Can you work these out from the model? Positions are in its coordinate system, mm. A direction names the side the tool comes from. Give positions to 0.01 mm unless a question says otherwise; leave off trailing zeros. Order: outer loops, then holes, each group sorted by start corner. A loop starts at its lowest first (then second) coordinate and runs counter-clockwise, first axis right, second up. Notation, with made-up numbers: (-30, 76) - (-3, 76) arc R25 cw to (-3, 93) - close; hole circle Ø11 at (45.5, 35.25). An arc over 180 degrees is marked (long way). Answer as a JSON object with one key per item and string values.
```python
from build123d import *

# Parameters (mm, degrees)
F0_W     = 40
F0_H     = 16
F0_W_2   = 32
F0_H_2   = 8
F1_DEPTH = 2.5
F2_R     = 2
F4_DEPTH = 12.5


with BuildPart() as f1:
    # F0 (on Top) → F1 (new body, symmetric)
    with BuildSketch(Plane.XY):
        Rectangle(F0_W, F0_H)
        Rectangle(F0_W_2, F0_H_2, mode=Mode.SUBTRACT)
    extrude(amount=F1_DEPTH, both=True)

    # F2
    f2_edges = [f1.edges().sort_by_distance(p)[0] for p in [
        (-20, 8, 0),
        (-20, -8, 0),
        (20, -8, 0),
        (20, 8, 0),
    ]]
    fillet(f2_edges, radius=F2_R)

    # F3 (on face) → F4 (cut, symmetric)
    with BuildSketch(Plane.XY.offset(2.5)):
        Polygon((16, 0), (16, -2.256422), (20, 0.861545), (20, 2.871813), align=None)
    extrude(amount=F4_DEPTH, both=True, mode=Mode.SUBTRACT)


solid = f1.part
```
Q1. Which directions (+Z, -Z, +X, -X, +Y, -Y) give clear straight access to the entire face, cutting with the end or side of a thin tool? Please do faces 1 (the face through (17.97, -0.72, 0.04)), 2 (the face through (0, 5, -2.5)).
Recorded:
{"face 1": "+Z, -Z", "face 2": "-Z, +X, -X, +Y, -Y"}
Q2. I need wall thicknesses on L1, parallel to Y at x = -2, z = 1.95; L2, parallel to X at y = 0.5, z = -0.85; L3, parallel to X at y = -1.5, z = -1.9. Which ranges of each line are inside material? Lowest first, please.
Recorded:
{"L1": "y = -8 to -4, 4 to 8", "L2": "x = -20 to -16, 16 to 16.7, 19.54 to 20", "L3": "x = -20 to -16, 16.97 to 20"}
Q3. If we section it at B-B, the plane x = 16.5: Please give me the cut outline in (y, z).
Recorded:
{"outline": "(-8, -2.5) - (-1.87, -2.5) - (-1.87, 2.5) - (-8, 2.5) - close; (0.36, -2.5) - (8, -2.5) - (8, 2.5) - (0.36, 2.5) - close"}
Q4. If we section it at A-A, the plane y = -3.25: Please give me the cut outline in (x, z).
Recorded:
{"outline": "(-20, -2.5) - (-16, -2.5) - (-16, 2.5) - (-20, 2.5) - close; (16, -2.5) - (20, -2.5) - (20, 2.5) - (16, 2.5) - close"}
Q5. I'm going to push a flat-ended pin straight in: pin 1 Ø6 at (x, y) = (-6.5, -2.5) entering from -Z. Where does the tip first touch, or does it pass through?
Recorded:
{"pin 1": "stops at z = -2.5"}
Q6. If we section it at C-C, the plane z = -1.85: Please give me the cut outline in (x, y).
Recorded:
{"outline": "(-20, -6) arc R2 ccw to (-18, -8) - (18, -8) arc R2 ccw to (20, -6) - (20, 0.86) - (16, -2.26) - (16, -4) - (-16, -4) - (-16, 4) - (16, 4) - (16, 0) - (20, 2.87) - (20, 6) arc R2 ccw to (18, 8) - (-18, 8) arc R2 ccw to (-20, 6) - close"}
Q7. We'd pull the mould along Y, two halves only. Please class faces 3 (the face through (-19.43, -7.4, 0.04)), 4 (the face through (20, -3, 0)), 5 (the face through (-16, 0, 0)): released by +Y, released by -Y, zero draft, split by the parting line, or undercut.
Recorded:
{"face 3": "released by -Y", "face 4": "zero draft", "face 5": "undercut"}
